from build123d import *

# Parameters (mm, degrees)
F0_W     = 26.4738108963
F0_H     = 8.0572450534
F2_R     = 7.9422363179
F3_DEPTH = 26.4738108963
F5_R     = 2.1448281624
F5_R_2   = 2.5012779103
F5_R_3   = 2.6092964081
F5_R_4   = 2.5232516324
F5_R_5   = 2.8839759477
F5_R_6   = 2.7467200302
F6_DEPTH = 5.3714960814


with BuildPart() as f1:
    # F0 (on Front) → F1 (revolve)
    with BuildSketch(Plane.XZ):
        Polygon((-48.3434833586, 37.6964099705), (-48.3434833586, 22.5411076099), (-21.8696724623, 22.5411076099), (-21.8696724623, 30.2146784961), (-42.9719872773, 30.2146784961), (-42.9719872773, 37.6964099705), align=None)
        with Locations((-35.1065779105, 18.5124850832)):
            Rectangle(F0_W, F0_H)
    revolve(axis=Axis((-35.1065779105, 0, 14.4838625565), (1, 0, 0)))

    # F2 (on face) → F3 (cut, through all)
    with BuildSketch(Plane.YZ.offset(-21.8696724623)):
        with Locations((0, 14.4838625565)):
            Circle(F2_R)
    extrude(amount=-F3_DEPTH, mode=Mode.SUBTRACT)

    # F5 (on face) → F6 (cut, through all)
    with BuildSketch(Plane.YZ.offset(-42.9719872773)):
        with Locations((-9.5919603482, 32.5167477131)):
            Circle(F5_R)
        with Locations((9.2082852498, 32.7085889876)):
            Circle(F5_R_2)
        with Locations((-9.5919603482, -3.3571864478)):
            Circle(F5_R_3)
        with Locations((9.2082852498, -3.3571864478)):
            Circle(F5_R_4)
        with Locations((-19.7594407946, 14.8675395176)):
            Circle(F5_R_5)
        with Locations((19.7594407946, 14.8675395176)):
            Circle(F5_R_6)
    extrude(amount=-F6_DEPTH, mode=Mode.SUBTRACT)


solid = f1.part
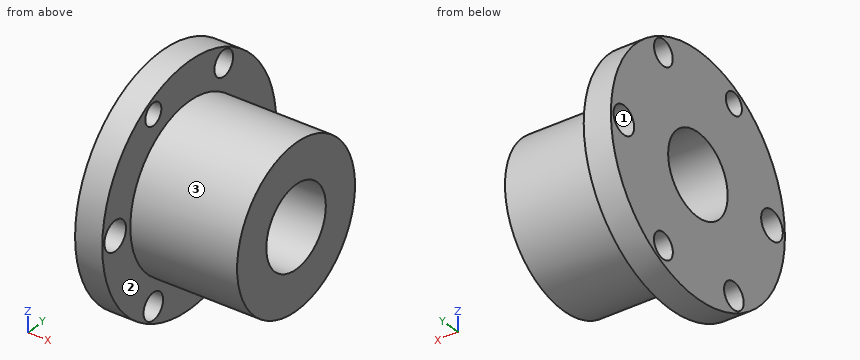
The listing builds one solid part. Answer for the finished solid, in the listing's coordinates (mm). Face numbers are marked on the shaded views. Give positions to 0.01 mm unless a question says otherwise; leave off trailing zeros. Order: outer loops, then holes, each group sorted by start corner. A loop starts at its lowest first (then second) coordinate and runs counter-clockwise, first axis right, second up. Notation, with made-up numbers: (10, 44) - (55, 44) arc R30 ccw to (55, 66) - close; hole circle Ø2 at (5.5, -1). An arc over 180 degrees is marked (long way). One line per item, written item: value. Start each with the question number.
1) A cutting plane is placed at A-A on y = 0. Give the vertices of the cut face in (x, z), then the cut area to 3 significant figures.
2) A cutting plane is placed at C-C on y = 9.5. Give the vertices of the cut face in (x, z), then the cut area to 3 significant figures.
3) Find the intervals of material crossed by L1, parallel to Z at x = -28, y = 0; L2, parallel to Y at x = -45.5, z = 14.5; L3, parallel to Y at x = -43.5, z = 15.5, in increasing order.
4) The mould has two halves that part along Z. Classify the marked faces 1, 2 and 3: released by +Z, released by -Z, zero draft, split by the parting line, or undercut.
5) Given pin 1 Ø1 at (x, z) = (-34.5, 12) entering from -Y; pin 2 Ø4.5 at (y, z) = (-19.76, 14.87) entering from -X; pin 3 Ø2 at (x, z) = (-28.5, 6) entering from +Y; pin 4 Ø5 at (x, z) = (-29.5, 30.5) entering from +Y, each flat-ended and moving along its own axis, determine where each tip first touches the part or whether it passes through.
6) A cutting plane is placed at D-D on x = -45.5. Give the vertices of the cut face in (y, z).
7) A cutting plane is placed at B-B on z = 8. Give the vertices of the cut face in (x, y), then the cut area to 3 significant figures.
Answer sheet:
1. outline: (-48.34, -8.73) - (-42.97, -8.73) - (-42.97, -1.25) - (-21.87, -1.25) - (-21.87, 6.54) - (-48.34, 6.54) - close; (-48.34, 22.43) - (-21.87, 22.43) - (-21.87, 30.21) - (-42.97, 30.21) - (-42.97, 37.7) - (-48.34, 37.7) - close
1. area: 493 mm2
2. outline: (-48.34, -6.7) - (-42.97, -6.7) - (-42.97, -5.86) - (-48.34, -5.86) - close; (-48.34, -0.85) - (-42.97, -0.85) - (-42.97, 1.95) - (-21.87, 1.95) - (-21.87, 27.02) - (-42.97, 27.02) - (-42.97, 30.22) - (-48.34, 30.22) - close; (-48.34, 35.19) - (-42.97, 35.19) - (-42.97, 35.66) - (-48.34, 35.66) - close
2. area: 703 mm2
3. L1: z = -1.25 to 6.54, 22.43 to 30.21
3. L2: y = -23.21 to -22.62, -16.9 to -7.94, 7.94 to 17.04, 22.48 to 23.21
3. L3: y = -23.19 to -22.57, -16.95 to -7.88, 7.88 to 17.09, 22.43 to 23.19
4. face 1: undercut
4. face 2: zero draft
4. face 3: split by the parting line
5. pin 1: stops at y = -15.61
5. pin 2: passes through
5. pin 3: stops at y = 13.84
5. pin 4: stops at y = 8.05
6. outline: circle Ø46.43 at (0, 14.48); hole circle Ø5.77 at (-19.76, 14.87); hole circle Ø5.22 at (-9.59, -3.36); hole circle Ø4.29 at (-9.59, 32.52); hole circle Ø15.88 at (0, 14.48); hole circle Ø5.05 at (9.21, -3.36); hole circle Ø5 at (9.21, 32.71); hole circle Ø5.49 at (19.76, 14.87)
7. outline: (-48.34, -22.29) - (-42.97, -22.29) - (-42.97, -14.33) - (-21.87, -14.33) - (-21.87, -4.59) - (-48.34, -4.59) - close; (-48.34, 4.59) - (-21.87, 4.59) - (-21.87, 14.33) - (-42.97, 14.33) - (-42.97, 22.29) - (-48.34, 22.29) - close
7. area: 601 mm2
